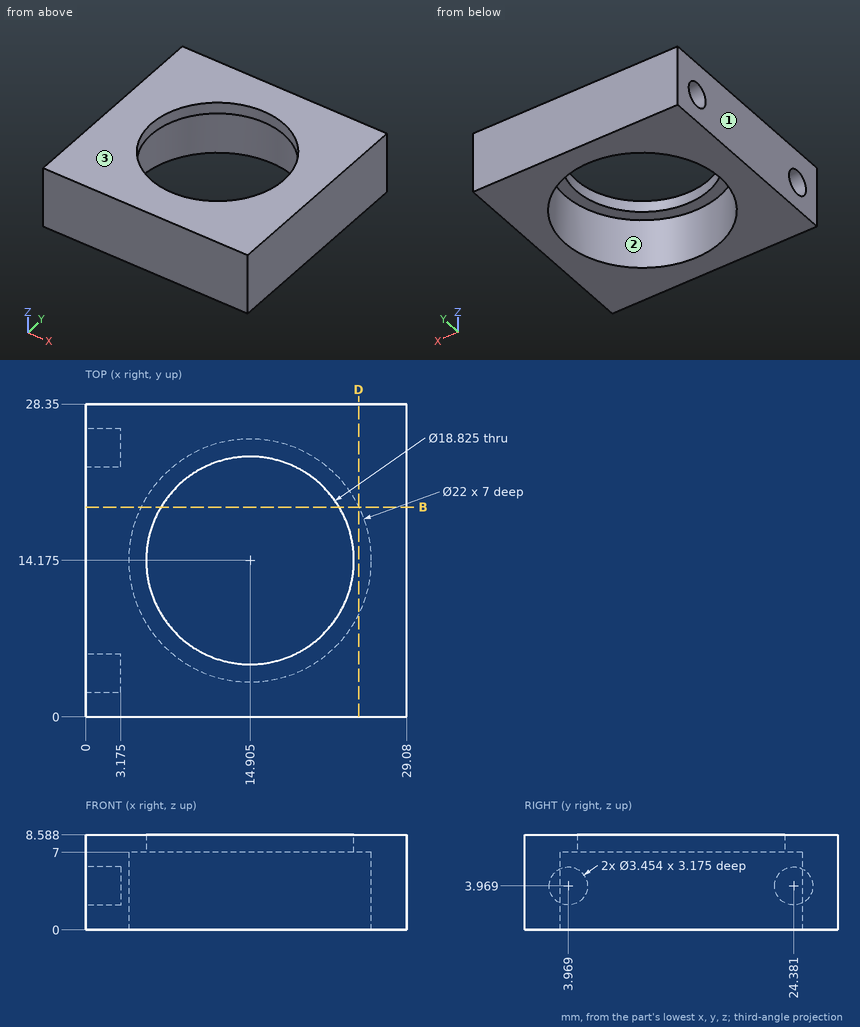
Here's the drawing with two shaded views (mm, measured from the low corner). I have some questions. Round coordinates to 2 decimals unless told otherwise and drop trailing zeros. Loops run counter-clockwise (first coordinate to the right, second up) from the corner with the lowest first, then second, coordinate; pieces in that order, holes last. Notation, with made-up numbers: M 31.25,58 L 75.25,58 A6 ccw 75.25,66 Z; hole C 80,69 d1. An arc over 180 degrees is marked long. Answer as a JSON object with one key per item and string values. Group by question number.
Q1. We'd pull the mould along X, two halves only. Please class the marked faces 1, 2 and 3: +X half, -X half, draft (parallel to the pull), parting line (faces both ways), or undercut.
Q2. Will this pin go through, and if not, where does the flat tip stop? pin 1 (2 mm diameter, centred on y = 24.38, z = 3.97, fed in from -X) (1 decimal).
Q3. Imagine slicing it at D-D, the plane x = 24.75. Please give me the cut outline in (y, z), then the cut area to 3 significant figures.
Q4. Imagine slicing it at B-B, the plane y = 19. Please give me the cut outline in (x, z).
Q5. Please list where these lines run through material, in increasing order: L1, parallel to X at y = 25.5, z = 5.25 (1 decimal); L2, parallel to X at y = 21.5, z = 6; L3, parallel to Y at x = 19.5, z = 0.75.
Findings:
{
 "1": {"face 1": "-X half", "face 2": "undercut", "face 3": "draft"},
 "2": {"pin 1": "stops at x = 3.2"},
 "3": {"outline": "M 0,0 L 9.27,0 L 9.27,7 L 19.08,7 L 19.08,0 L 28.35,0 L 28.35,8.59 L 0,8.59 Z", "area": "175 mm2"},
 "4": {"outline": "M 0,0 L 5.02,0 L 5.02,7 L 6.82,7 L 6.82,8.59 L 0,8.59 Z; M 22.99,7 L 24.79,7 L 24.79,0 L 29.08,0 L 29.08,8.59 L 22.99,8.59 Z"},
 "5": {"L1": "x = 3.2 to 29.1", "L2": "x = 0 to 6.7, 23.11 to 29.08", "L3": "y = 0 to 4.18, 24.17 to 28.35"}
}
